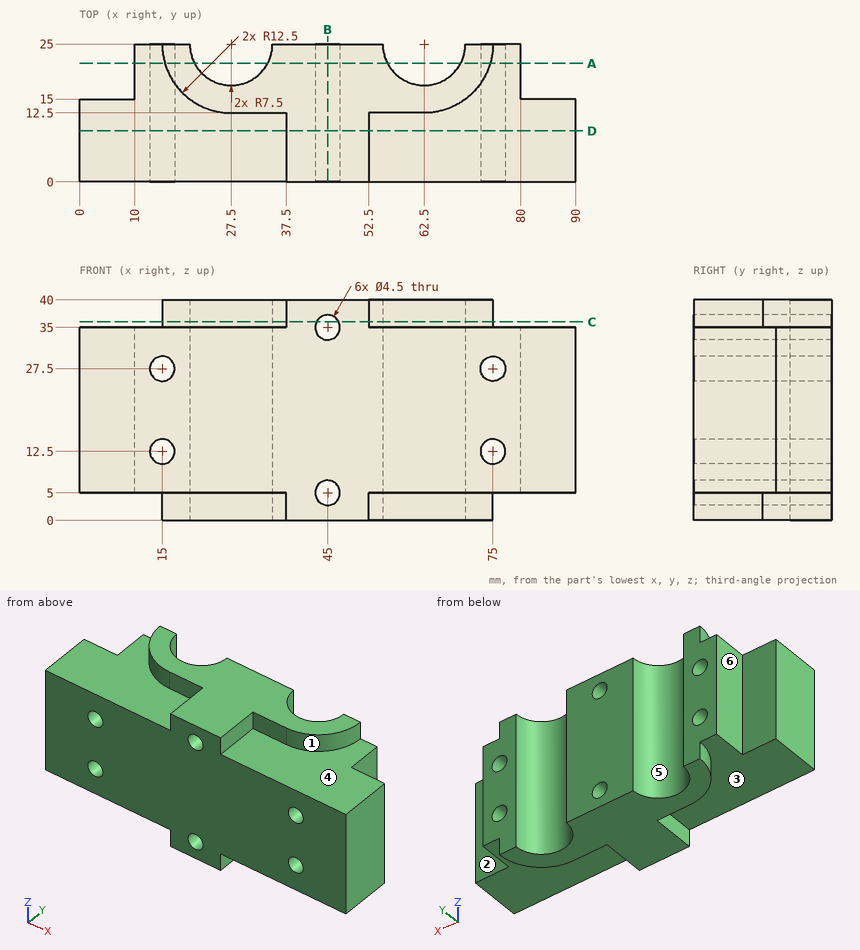
Job drawing, mm, ordinate dimensions from the low corner. One solid piece. A direction names the side the tool comes from. Coordinates: 2 decimals unless noted, no trailing zeros. Order: outer loops, then holes, each group sorted by start corner. A loop starts at its lowest first (then second) coordinate and runs counter-clockwise, first axis right, second up. Notation, with made-up numbers: M 19.5,78 L 39.5,78 A29 cw 39.5,107 Z; hole C -34.5,40.25 d6. An arc over 180 degrees is marked long. Answer as CSV lines item,"result".
(1) Pull direction X, two halves, no side cores. Call the marked faces 4, 5 and 6: +X half, -X half, draft (parallel to the pull), parting line (faces both ways), or undercut.
Geometry says:
face 4,"draft"
face 5,"undercut"
face 6,"-X half"
(2) Band-saw the part on B-B, the plane x = 45. List the corners of the cut face in (y, z), then the cut area to 3 significant figures.
Geometry says:
outline,"M 0,0 L 25,0 L 25,2.75 L 0,2.75 Z; M 0,7.25 L 25,7.25 L 25,32.75 L 0,32.75 Z; M 0,37.25 L 25,37.25 L 25,40 L 0,40 Z"
area,"775 mm2"
(3) 3-axis set-ups, long thin cutter, end or side, ignore diameter. For the marked faces 1, 2 and 3: which of +Z, -Z, +X, -X, +Y, -Y reach the whole face in a straight line?
Geometry says:
face 1,"+Z, +X, -Y"
face 2,"+Z, -Z, +X, +Y"
face 3,"-Z, -X, -Y"
(4) Band-saw the part on A-A, the plane y = 21.5. State how many separate pieces and enclosed holes the cut face has, then the cut area to 3 significant figures.
Geometry says:
separate pieces,"3"
enclosed holes,"6"
area,"1,530 mm2"
(5) Band-saw the part on C-C, the plane z = 36. List the corners of the cut face in (x, y).
Geometry says:
outline,"M 15,25 A12.5 ccw 27.5,12.5 L 37.5,12.5 L 37.5,0 L 42.98,0 L 42.98,25 L 35,25 A7.5 cw 20,25 Z; M 47.02,0 L 52.5,0 L 52.5,12.5 L 62.5,12.5 A12.5 ccw 75,25 L 70,25 A7.5 cw 55,25 L 47.02,25 Z"
(6) Flat gauge pins, fed straight in: pin 1 (4 mm diameter, centred on y = 5, z = 2, fed in from +X); pin 2 (1.5 mm diameter, centred on x = 55.5, z = 36.5, fed in from -Y); pin 3 (7.5 mm diameter, centred on x = 15.5, y = 12.5, fed in from -Z). Where does each tip first touch, or does it go through?
Geometry says:
pin 1,"stops at x = 52.5"
pin 2,"stops at y = 12.5"
pin 3,"stops at z = 5"
(7) Wall check: line 1 along Z through (x, y) = (45, 15); line 2 along Z through (x, y) = (75, 6); line 3 along X through (y, z) = (22.25, 23). Give the ranges that are in metal, low to high.
Geometry says:
line 1,"z = 0 to 2.75, 7.25 to 32.75, 37.25 to 40"
line 2,"z = 5 to 10.25, 14.75 to 25.25, 29.75 to 35"
line 3,"x = 10 to 20.52, 34.48 to 55.52, 69.48 to 80"
(8) Band-saw the part on D-D, the plane y = 9.25. List the corners of the cut face in (x, z), then the cut area to 3 significant figures.
Geometry says:
outline,"M 0,5 L 37.5,5 L 37.5,0 L 52.5,0 L 52.5,5 L 90,5 L 90,35 L 52.5,35 L 52.5,40 L 37.5,40 L 37.5,35 L 0,35 Z; hole C 15,12.5 d4.5; hole C 15,27.5 d4.5; hole C 45,5 d4.5; hole C 45,35 d4.5; hole C 75,12.5 d4.5; hole C 75,27.5 d4.5"
area,"2,750 mm2"
